Check sheet for the modelled part. Datum: model origin and axes. Units: mm. Face numbers are marked on the shaded views. A direction names the side the tool comes from. Give positions to 0.01 mm unless a question says otherwise; leave off trailing zeros. Order: outer loops, then holes, each group sorted by start corner. A loop starts at its lowest first (then second) coordinate and runs counter-clockwise, first axis right, second up. Notation, with made-up numbers: (65.5, -9) -> (76.5, -9) arc R26 ccw to (76.5, 29) -> close; hole circle Ø8 at (66.5, 26). An arc over 180 degrees is marked (long way). Write each question's results on one line, items separated by ' | '.
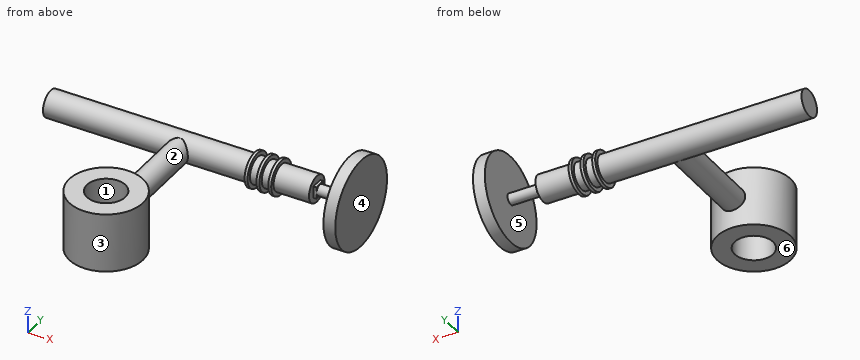
from build123d import *

# Parameters (mm, degrees)
SKETCH2_R           = 6.25
EXTRUDE1_DEPTH      = 5
SKETCH3_R           = 2
EXTRUDE2_DEPTH      = 22.5
EXTRUDE3_DEPTH      = 22.5
EXTRUDE3_DEPTH_BACK = 22.5
SKETCH4_R           = 2.25
SKETCH5_R           = 2.933820517
EXTRUDE4_DEPTH      = 0.5
LPATTERN1_COUNT     = 3
LPATTERN1_PITCH     = 2
SKETCH9_W           = 2
SKETCH9_H           = 2
EXTRUDE6_DEPTH      = 0.5
SKETCH7_R           = 3.25
CUT_EXTRUDE1_DEPTH  = 36.719451677
SKETCH6_R           = 0.925
EXTRUDE7_DEPTH      = 5
SKETCH10_R          = 7.5
EXTRUDE8_DEPTH      = 2


with BuildPart() as part:
    # Sketch2 → Extrude1 (new, symmetric)
    with BuildSketch(Plane.XY):
        Circle(SKETCH2_R)
    extrude(amount=EXTRUDE1_DEPTH, both=True)

    # Sketch3 → Extrude2 (add)
    with BuildSketch(Plane(origin=(0, 0, 0), x_dir=(-1, 0, 0), z_dir=(0, 1, 0))):
        with Locations(Location((0, 0, 0), (0, 0, 270))):
            Circle(SKETCH3_R)
    extrude(amount=EXTRUDE2_DEPTH)

    # Sketch4 → Extrude3 (add, two sides: drawn at the far end of the back side and taken through both)
    with BuildSketch(Plane(origin=(0, 0, 0), x_dir=(0, 0, -1), z_dir=(1, 0, 0)).offset(-EXTRUDE3_DEPTH_BACK)):
        with Locations((0, 22.5)):
            Circle(SKETCH4_R)
    extrude(amount=EXTRUDE3_DEPTH + EXTRUDE3_DEPTH_BACK)

    # Sketch5 → Extrude4 (add)
    with BuildSketch(Plane(origin=(12, 0, 0), x_dir=(0, 0, -1), z_dir=(1, 0, 0))):
        with Locations((0, 22.5)):
            Circle(SKETCH5_R)
    extrude4 = extrude(amount=EXTRUDE4_DEPTH)

    # LPattern1: Extrude4 ×3
    with Locations(*[(i * LPATTERN1_PITCH, 0, 0) for i in range(1, LPATTERN1_COUNT)]):
        add(extrude4)

    # Sketch9 → Extrude6 (add)
    with BuildSketch(Plane(origin=(22.5, 0, 0), x_dir=(0, 0, -1), z_dir=(1, 0, 0))):
        with Locations((0, 22.5)):
            Rectangle(SKETCH9_W, SKETCH9_H)
    extrude(amount=EXTRUDE6_DEPTH)

    # Sketch7 → Cut-Extrude1 (cut, through all)
    with BuildSketch(Plane.XY.offset(5)):
        Circle(SKETCH7_R)
    extrude(amount=-CUT_EXTRUDE1_DEPTH, mode=Mode.SUBTRACT)

    # Sketch6 → Extrude7 (add)
    with BuildSketch(Plane(origin=(23, 0, 0), x_dir=(0, 0, -1), z_dir=(1, 0, 0))):
        with Locations((0, 22.5)):
            Circle(SKETCH6_R)
    extrude(amount=EXTRUDE7_DEPTH)

    # Sketch10 → Extrude8 (add)
    with BuildSketch(Plane(origin=(28, 0, 0), x_dir=(0, 0, -1), z_dir=(1, 0, 0))):
        with Locations((0, 22.5)):
            Circle(SKETCH10_R)
    extrude(amount=EXTRUDE8_DEPTH)


solid = part.part
1. Material ranges on probe 1 along Y at (x, z) = (0, 0.75); probe 2 along X at (y, z) = (19, -6.5); probe 3 along X at (y, z) = (7, 0), recorded low to high. Write a range as from..to.
Verdict:
probe 1: y = -6.25..-3.25, 3.25..24.62 | probe 2: x = 28..30 | probe 3: x = -2..2
2. Section check D-D on y = 18. Record the cut outline in (x, z).
Verdict:
outline: circle Ø4 at (0, 0); (28, -6) -> (30, -6) -> (30, 6) -> (28, 6) -> close
3. Section check A-A on x = 0. Record the cut outline in (y, z).
Verdict:
outline: (-6.25, -5) -> (-3.25, -5) -> (-3.25, 5) -> (-6.25, 5) -> close; (3.25, -5) -> (6.25, -5) -> (6.25, -2) -> (21.47, -2) arc R2.25 ccw (long way) to (21.47, 2) -> (6.25, 2) -> (6.25, 5) -> (3.25, 5) -> close
4. Mould release check, pull along X, two halves, no side actions. Record for the marked faces 3, 4, 5 and 6: +X half, -X half, draft (parallel to the pull), parting line (faces both ways), or undercut.
Verdict:
face 3: parting line | face 4: +X half | face 5: undercut | face 6: draft
5. Gauge pin test, flat ends, axial feed: pin 1 Ø6 at (x, y) = (-4.5, 10.5) entering from +Z; pin 2 Ø3 at (x, z) = (14, -1.5) entering from -Y; pin 3 Ø0.6 at (x, y) = (22.5, 22) entering from -Z. Record the tip position at first contact, or that the pin passes through.
Verdict:
pin 1: stops at z = 1.32 | pin 2: stops at y = 19.57 | pin 3: stops at z = -2.24
6. Section check B-B on y = 0. Record the cut outline in (x, z), then the cut area to 3 significant figures.
Verdict:
outline: (-6.25, -5) -> (-3.25, -5) -> (-3.25, 5) -> (-6.25, 5) -> close; (3.25, -5) -> (6.25, -5) -> (6.25, 5) -> (3.25, 5) -> close | area: 60.0 mm^2
7. Access from +Z, -Z, +X, -X, +Y, -Y to the whole of each face (thin tool, end or side, straight path). Record for the marked faces 1 and 2.
Verdict:
face 1: +Z, -Z | face 2: none
8. Section check C-C on z = 6. Record the cut outline in (x, y), then the cut area to 3 significant figures.
Verdict:
outline: (28, 18) -> (30, 18) -> (30, 27) -> (28, 27) -> close | area: 18.0 mm^2
